Job drawing, mm, ordinate dimensions from the low corner. One solid piece. A direction names the side the tool comes from. Coordinates: 2 decimals unless noted, no trailing zeros. Write each loop counter-clockwise with the first axis right and the second up, starting at its lowest first coordinate (ties: lowest second). Pieces come first, ordered by that corner, then holes. Notation, with made-up numbers: (88.5, 6) - (118.5, 6) arc R15 cw to (118.5, 32) - close; hole circle Ø3 at (46, 13.25). An arc over 180 degrees is marked (long way). Use a Markdown table: item, result.
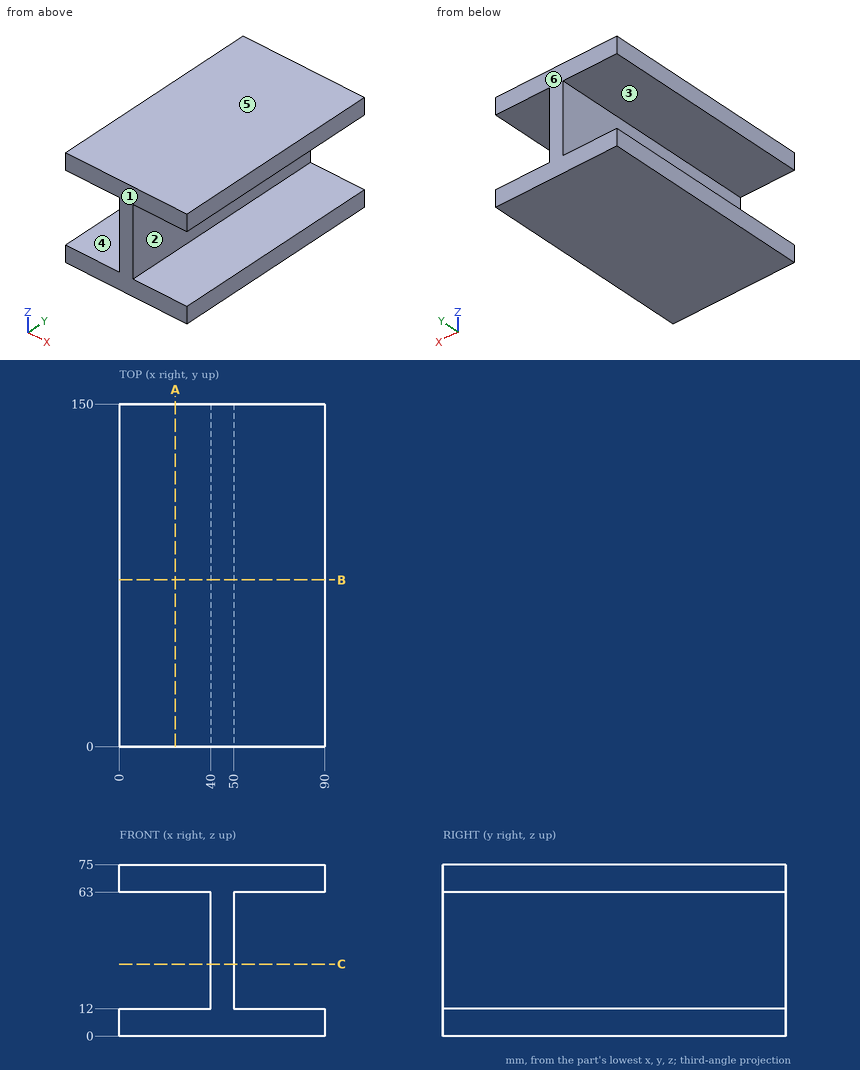
Item 1: Two-plate mould, pull along Z, no slides. Class the marked faces 4, 5 and 6: pulls with the +Z half, pulls with the -Z half, needs draft (parallel to the pull), parting line crosses it, or undercut.
From the geometry:
| item | result |
|---|---|
| face 4 | undercut |
| face 5 | pulls with the +Z half |
| face 6 | needs draft |
Item 2: Band-saw the part on B-B, the plane y = 73. Give the cut face in (x, z).
From the geometry:
| item | result |
|---|---|
| outline | (0, 0) - (90, 0) - (90, 12) - (50, 12) - (50, 63) - (90, 63) - (90, 75) - (0, 75) - (0, 63) - (40, 63) - (40, 12) - (0, 12) - close |
Item 3: Band-saw the part on A-A, the plane x = 24.5. Give the cut face in (y, z).
From the geometry:
| item | result |
|---|---|
| outline | (0, 0) - (150, 0) - (150, 12) - (0, 12) - close; (0, 63) - (150, 63) - (150, 75) - (0, 75) - close |
Item 4: Band-saw the part on C-C, the plane z = 31.5. Give the cut face in (x, y), then the cut area to 3 significant figures.
From the geometry:
| item | result |
|---|---|
| outline | (40, 0) - (50, 0) - (50, 150) - (40, 150) - close |
| area | 1,500 mm^2 |
Item 5: Drop flat-ended pins along their axis: P1, Ø12, axis at y = 109, z = 44.5, coming from the +X side; P2, Ø10, axis at y = 29.5, z = 53, coming from the -X side. Give the stop position or say it passes through.
From the geometry:
| item | result |
|---|---|
| P1 | x = 50 |
| P2 | x = 40 |
Item 6: Which spindle directions (+Z, -Z, +X, -X, +Y, -Y) get a long thin tool onto all of the face, cutting with end or side? Do the marked faces 1, 2 and 3. Say none if no direction does.
From the geometry:
| item | result |
|---|---|
| face 1 | +Z, -Z, +X, -X, -Y |
| face 2 | +X, +Y, -Y |
| face 3 | -X, +Y, -Y |
Item 7: Drill centre lines: probe 1 along Z at (x, y) = (62, 84.5); probe 2 along X at (y, z) = (109.5, 18). Where is each one in solid material? Low to high.
From the geometry:
| item | result |
|---|---|
| probe 1 | 0 to 12, 63 to 75 |
| probe 2 | 40 to 50 |
